Build history of the part. All positions in model axes, mm. Give positions to 0.01 mm unless a question says otherwise; leave off trailing zeros. Loops run counter-clockwise (first coordinate to the right, second up) from the corner with the lowest first, then second, coordinate; pieces in that order, holes last. Notation, with made-up numbers: (-16.75, 22.25) -> (16.25, 22.25) arc R22 ccw to (16.25, 31.25) -> close; hole circle Ø5 at (23.25, 48.25). An arc over 180 degrees is marked (long way). Answer as a JSON object with one key per item and string values. Group by question number.
from build123d import *

# Parameters (mm, degrees)
SKETCH_1_W          = 94
SKETCH_1_H          = 63
EXTRUDE_1_DEPTH     = 37
FILLET_1_R          = 10
SKETCH_3_R          = 1.5
CUT_EXTRUDE_1_DEPTH = 10


with BuildPart() as part:
    # 草图1 → 凸台-拉伸1 (new body)
    with BuildSketch(Plane.XY):
        with Locations((-2.555555556, -0.5)):
            Rectangle(SKETCH_1_W, SKETCH_1_H)
    extrude(amount=EXTRUDE_1_DEPTH)

    # 圆角1
    fillet_1_edges = [part.edges().sort_by_distance(p)[0] for p in [
        (-49.555555556, 31, 18.5),
        (44.444444444, 31, 18.5),
        (44.444444444, -32, 18.5),
        (-49.555555556, -32, 18.5),
    ]]
    fillet(fillet_1_edges, radius=FILLET_1_R)

    # 草图3 → 切除-拉伸1 (cut)
    with BuildSketch(Plane.XY.offset(37)):
        with Locations((-39.555555556, -22)):
            Circle(SKETCH_3_R)
        with Locations((-39.555555556, 21)):
            Circle(SKETCH_3_R)
    extrude(amount=-CUT_EXTRUDE_1_DEPTH, mode=Mode.SUBTRACT)


solid = part.part
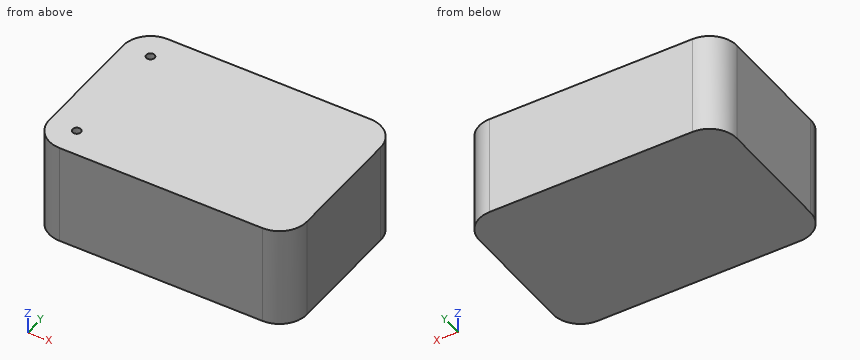
(1) Pin check, flat tip, straight feed: pin 1 (1.8 mm diameter, centred on x = -39.56, y = 21, fed in from +Z). Stop position of the tip, or through.
(2) Saw through at A-A on z = 33. List the corners of the cut face in (x, y), plus the area to 3 significant figures.
(3) Probe line 1 along X through (y, z) = (23, 29.5); line 2 along X through (y, z) = (-29, 4); line 3 along Y through (x, z) = (38, 29.5). List the from-to ranges inside material, lowest first. Write a range as [from, to].
Calculated:
{
 "1": {"pin 1": "stops at z = 27"},
 "2": {"outline": "(-49.56, -22) arc R10 ccw to (-39.56, -32) -> (34.44, -32) arc R10 ccw to (44.44, -22) -> (44.44, 21) arc R10 ccw to (34.44, 31) -> (-39.56, 31) arc R10 ccw to (-49.56, 21) -> close; hole circle Ø3 at (-39.56, -22); hole circle Ø3 at (-39.56, 21)", "area": "5,820 mm^2"},
 "3": {"line 1": "x = [-49.35, 44.24]", "line 2": "x = [-46.7, 41.59]", "line 3": "y = [-31.35, 30.35]"}
}
